Autodesk Inventor part; units mm, degrees
ref_plane "IDS_WORKPLANE{1}" through (0, 0, 0) normal (0, 1, 0) x (-1, 0, 0)
ref_plane "Work Plane3" through (7.1437, 0, 0) normal (0, 0, -1) x (1, 0, 0)
ref_plane "YZ Plane" through (0, 0, 0) normal (1, 0, 0) x (0, 1, 0)
sketch "Boceto1" plane through (0, 0, 0) normal (0, 0, 1) x (1, 0, 0)
  line L0 (0, 3.302) -> (1.905, 3.302)
  line L1 (1.905, 3.302) -> (3.175, 3.175)
  line L2 (3.175, 3.175) -> (11.1125, 3.175)
  line L3 (11.1125, 3.175) -> (11.1125, 2.4879)
  line L4 (11.1125, 2.4879) -> (11.1125, 0)
  line L5 (0, 3.9624) -> (0, -0.6604)
  line L6 (0, 3.302) -> (0, 0)
  line L7 (-0.4343, 0) -> (7.5114, 0)
  line L8 (-2.7437, 0) -> (13.4219, 0)
  line L9 (0, 0) -> (11.1125, 0)
  dimension "d0" = 0
  dimension "d1" = 7.9375
  dimension "d2" = 1.27
  dimension "d3" = 4.9759
  dimension "d4" = 6.35
  dimension "d5" = 6.604
  dimension "d6" = 11.1125
revolve "Cuerpo" add sketch "Boceto1" angle 360 about axis through (-0.4343, 0, 0) along (1, 0, 0)
sketch "Boceto2" plane through (0, 0, 0) normal (-1, 0, 0) x (0, 0, 1)
  line L0 (-6.35, 3.556) -> (6.35, 3.556)
  line L1 (6.35, 3.556) -> (6.35, -3.556)
  line L2 (6.35, -3.556) -> (-6.35, -3.556)
  line L3 (-6.35, -3.556) -> (-6.35, 3.556)
  line L4 (-8.89, 0) -> (8.89, 0)
  line L5 (0, 4.9784) -> (0, -4.9784)
  dimension "d7" = 3.556
  dimension "d8" = 7.112
  dimension "d9" = 6.35
  dimension "d10" = 12.7
extrude "Cabeza" add sketch "Boceto2" along normal blind 5.1816
ref_plane "IDS_WORKPLANE{1}" through (0, 0, 0) normal (0, 1, 0) x (-1, 0, 0)
sketch "Boceto3" plane through (0, 0, 0) normal (0, 1, 0) x (-1, 0, 0)
  arc A0 (5.1816, 0) -> (-0.1952, 9.525) centre (-5.9436, 0) ccw
  line L0 (0, -9.6663) -> (0, 13.5477)
  line L1 (8.9083, 0) -> (-8.4189, 0)
  line L2 (5.1816, 6.35) -> (5.1816, 9.525)
  line L3 (5.1816, 9.525) -> (-0.1952, 9.525)
  line L4 (5.1816, 6.35) -> (5.1816, -6.35)
  dimension "d15" = 11.1252
  dimension "d19" = 19.05
revolve "Empalme1" cut sketch "Boceto3" angle 360 about axis through (-10, 0, 0) along (1, 0, 0) contours A0 L0 L3 L2 L4 | A0 L3 L0
thread "Rosca"
ref_plane "Work Plane3" through (7.1437, 0, 0) normal (0, 0, -1) x (1, 0, 0)
equation "\"d7\" = 0.5 * KBR"
equation "\"d8\" = KBR"
equation "\"d9\" = 0.5 * KOL"
equation "\"d10\" = KOL"
equation "\"d11\" = KOH"
equation "\"d15\" = KR"
equation "\"d19\" = 1.5 * KOL"
equation "\"d1\" = GEL"
equation "\"d2\" = GAL"
equation "\"d3\" = SPD"
equation "\"d4\" = GD"
equation "\"d5\" = BDM"
equation "\"d6\" = NLG"
equation "\"GD\" = NND"
equation "\"NLG\" = 11.1125"
equation "\"GAL\" = 1.27"
equation "\"GEL\" = 7.9375"
equation "\"BDM\" = 6.604"
equation "\"KOL\" = 12.7"
equation "\"KBR\" = 7.112"
equation "\"KOH\" = 5.1816"
equation "\"KR\" = 11.1252"
equation "\"SPD\" = GD1"
equation "\"RR\" = -0.5 * BDM + 0.5 * KBR"
equation "\"d13\" = 0.5 * KOL"
equation "\"GUL\" = 0"
equation "\"PHH\" = 0.15 * KOH"
equation "\"THREADDIA\" = 6.35"
equation "\"TOA\" = 30deg"
equation "\"NND\" = 6.35"
equation "\"GD1\" = 4.97586"
properties part number "ANSI/ASME B18.5 - 1/4 - 20 - 7/16" material "Acero, suave"
Verification items for the finished model (mm, model axes). A direction names the side the tool comes from. Give positions to 0.01 mm unless a question says otherwise; leave off trailing zeros. Order: outer loops, then holes, each group sorted by start corner. A loop starts at its lowest first (then second) coordinate and runs counter-clockwise, first axis right, second up. Notation, with made-up numbers: M 87,-36 L 127,-36 A23 ccw 127,-5 Z; hole C -30,70.5 d2. An arc over 180 degrees is marked long. Return JSON: item names as keys, results as strings. Group by question number.
1) Go/stop test with flat-tipped pins: pin 1 Ø6 at (x, z) = (6.5, 1.5) entering from +Y (3 decimals); pin 2 Ø6 at (x, z) = (6.5, -4) entering from +Y; pin 3 Ø4 at (x, y) = (3.5, 1) entering from -Z. Record where each tip stops, or that it passes through.
2) Section check A-A on x = 6.25. Record the cut outline in (y, z) (3 decimals).
3) Section check B-B on x = 1.25. Record the cut outline in (y, z).
4) Access from +Z, -Z, +X, -X, +Y, -Y to the whole of each face (thin tool, end or side, straight path). Record for faces 1 (the face through (-2, -3.556, 0)), 2 (the face through (7.2, -0.69, -3.1)).
5) Scan lines: line 1 (Z direction, x = 1, y = -0.25); line 2 (X direction, y = -3, z = -4.75); line 3 (X direction, y = -1, z = -0.75). Record each from-to range of solid material in increasing order.
Answer block:
{
 "1": {"pin 1": "stops at y = 3.175", "pin 2": "stops at y = 3.01", "pin 3": "stops at z = -3.3"},
 "2": {"outline": "C 0,0 d6.35"},
 "3": {"outline": "C 0,0 d6.6"},
 "4": {"face 1": "+Z, -Z, +X, -X, -Y", "face 2": "+X"},
 "5": {"line 1": "z = -3.29 to 3.29", "line 2": "x = -3.66 to 0", "line 3": "x = -5.11 to 11.11"}
}
